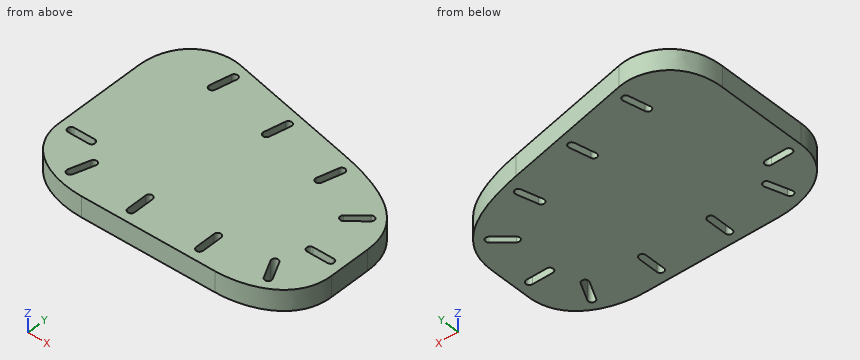
from build123d import *

# Parameters (mm, degrees)
EXTRUDE_1_DEPTH       = 10
CUT_EXTRUDE_1_DEPTH   = 149.427210809
PATTERN_CURVE_1_DEPTH = 10


# Read off the part's stored shape, not the designer's step: Кривая1
with BuildPart() as part:
    # Эскиз1_fr → Бобышка-Вытянуть1 (new body)
    with BuildSketch(Plane.XY):
        with BuildLine():
            Line((0, 0), (0, 20))
            add(Edge.make_bspline(
                [(0, 20), (0, 38.146025899), (-14.209474182, 48.611098897), (-41.986949672, 54.649680525)],
                knots=[0, 0, 0, 0, 1, 1, 1, 1], degree=3))
            Line((-41.986949672, 54.649680525), (-103.301225383, 67.978870897))
            add(Edge.make_bspline(
                [(-103.301225383, 67.978870897), (-115.500001367, 70.63077872), (-131.292525164, 63.393306184), (-131.292525164, 43.097715536)],
                knots=[0, 0, 0, 0, 1, 1, 1, 1], degree=3))
            Line((-131.292525164, 43.097715536), (-131.292525164, 0))
            add(Edge.make_bspline(
                [(-97.969549234, -25.769768053), (-112.011160689, -25.769768053), (-131.292525164, -19.025155818), (-131.292525164, 0)],
                knots=[0, 0, 0, 0, 1, 1, 1, 1], degree=3))
            Line((-97.969549234, -25.769768053), (-33.545129103, -25.769768053))
            add(Edge.make_bspline(
                [(-33.545129103, -25.769768053), (-19.444866568, -25.769768053), (0, -19.063757455), (0, 0)],
                knots=[0, 0, 0, 0, 1, 1, 1, 1], degree=3))
        make_face()
    extrude(amount=EXTRUDE_1_DEPTH)

    # Эскиз2_fr → Вырез-Вытянуть1 (cut, through all)
    with BuildSketch(Plane(origin=(0, 0, 0), x_dir=(-1, 0, 0), z_dir=(0, 0, -1))):
        with BuildLine():
            Line((102.429251955, 61.832882372), (104.527789693, 52.179608775))
            ThreePointArc((104.527789693, 52.179608775), (103.259303337, 50.206407776), (101.286102339, 51.474894133))
            Line((101.286102339, 51.474894133), (99.1875646, 61.128167729))
            ThreePointArc((99.1875646, 61.128167729), (100.456050956, 63.101368728), (102.429251955, 61.832882372))
        make_face()
    extrude(amount=-CUT_EXTRUDE_1_DEPTH, mode=Mode.SUBTRACT)

    # Кривая1 outline → Кривая1 (cut)
    with BuildSketch(Plane.XY):
        with BuildLine():
            ThreePointArc((-66.925496948, 54.114674761), (-68.193983304, 56.08787576), (-70.167184303, 54.819389404))
            Line((-70.167184303, 54.819389404), (-72.265722041, 45.166115807))
            ThreePointArc((-72.265722041, 45.166115807), (-70.997235685, 43.192914809), (-69.024034687, 44.461401165))
            Line((-69.024034687, 44.461401165), (-66.925496948, 54.114674761))
        make_face()
        with BuildLine():
            ThreePointArc((-34.992445024, 46.929960503), (-36.164147849, 48.962124942), (-38.196312288, 47.790422117))
            Line((-38.196312288, 47.790422117), (-40.758641861, 38.249771252))
            ThreePointArc((-40.758641861, 38.249771252), (-39.586939036, 36.217606813), (-37.554774597, 37.389309638))
            Line((-37.554774597, 37.389309638), (-34.992445024, 46.929960503))
        make_face()
        with BuildLine():
            ThreePointArc((-9.659083383, 32.724100966), (-9.478152386, 35.062870683), (-11.816922103, 35.243801681))
            Line((-11.816922103, 35.243801681), (-19.320224464, 28.818071725))
            ThreePointArc((-19.320224464, 28.818071725), (-19.501155461, 26.479302007), (-17.162385743, 26.298371011))
            Line((-17.162385743, 26.298371011), (-9.659083383, 32.724100966))
        make_face()
        with BuildLine():
            ThreePointArc((-5.820481715, 4.607864038), (-4.161780443, 6.266565309), (-5.820481715, 7.925266581))
            Line((-5.820481715, 7.925266581), (-15.699224133, 7.925266581))
            ThreePointArc((-15.699224133, 7.925266581), (-17.357925405, 6.266565309), (-15.699224133, 4.607864038))
            Line((-15.699224133, 4.607864038), (-5.820481715, 4.607864038))
        make_face()
        with BuildLine():
            ThreePointArc((-17.811005152, -16.834920175), (-15.579870133, -17.559224215), (-14.855566092, -15.328089196))
            Line((-14.855566092, -15.328089196), (-19.342689651, -6.527221402))
            ThreePointArc((-19.342689651, -6.527221402), (-21.573824671, -5.802917361), (-22.298128711, -8.034052381))
            Line((-22.298128711, -8.034052381), (-17.811005152, -16.834920175))
        make_face()
        with BuildLine():
            ThreePointArc((-47.67905304, -19.949286338), (-46.020351768, -21.607987609), (-44.361650497, -19.949286338))
            Line((-44.361650497, -19.949286338), (-44.361650497, -10.070543919))
            ThreePointArc((-44.361650497, -10.070543919), (-46.020351768, -8.411842648), (-47.67905304, -10.070543919))
            Line((-47.67905304, -10.070543919), (-47.67905304, -19.949286338))
        make_face()
        with BuildLine():
            ThreePointArc((-80.694656818, -19.949286338), (-79.035955546, -21.607987609), (-77.377254274, -19.949286338))
            Line((-77.377254274, -19.949286338), (-77.377254274, -10.070543919))
            ThreePointArc((-77.377254274, -10.070543919), (-79.035955546, -8.411842648), (-80.694656818, -10.070543919))
            Line((-80.694656818, -10.070543919), (-80.694656818, -19.949286338))
        make_face()
        with BuildLine():
            ThreePointArc((-111.662441641, -17.601639491), (-110.581423079, -19.683460493), (-108.499602077, -18.602441931))
            Line((-108.499602077, -18.602441931), (-105.519357928, -9.18396559))
            ThreePointArc((-105.519357928, -9.18396559), (-106.60037649, -7.102144588), (-108.682197492, -8.18316315))
            Line((-108.682197492, -8.18316315), (-111.662441641, -17.601639491))
        make_face()
        with BuildLine():
            ThreePointArc((-125.472043449, 1.658701272), (-127.130744721, 0), (-125.472043449, -1.658701272))
            Line((-125.472043449, -1.658701272), (-115.593301031, -1.658701272))
            ThreePointArc((-115.593301031, -1.658701272), (-113.934599759, 0), (-115.593301031, 1.658701272))
            Line((-115.593301031, 1.658701272), (-125.472043449, 1.658701272))
        make_face()
    extrude(amount=PATTERN_CURVE_1_DEPTH, mode=Mode.SUBTRACT)


solid = part.part
Source: CAD feature listing. Evaluate the final solid. Frame: model axes, mm. Coordinates: 2 decimals unless noted, no trailing zeros. Loops run counter-clockwise (first coordinate to the right, second up) from the corner with the lowest first, then second, coordinate; pieces in that order, holes last. Notation, with made-up numbers: (87, 81.5) - (138, 81.5) arc R24 cw to (138, 91.5) - close; hole circle Ø4 at (-17, -2.75). An arc over 180 degrees is marked (long way). One line per item, written item: value. Start each with the question number.
1. Section B-B (x = -74.5). Return the cut outline in (y, z), and give its area (3 significant figures).
2. Section C-C (x = -93). Return the cut outline in (y, z), and give its area (3 significant figures).
3. Section A-A (z = 4.5). State how many separate pieces and enclosed holes the cut face has, and give its area (3 significant figures).
4. Contact query for flat-ended pins moving along their axis: P1, Ø3, axis at x = -119, z = 5, coming from the +Y side; P2, Ø5, axis at y = -16, z = 6, coming from the -X side; P3, Ø5, axis at y = -14, z = 3, coming from the +X side. Output: stop coordinate, or through.
5. Ray query, L1, parallel to X at y = -10, z = 0.5; L2, parallel to X at y = -9.5, z = 4; L3, parallel to X at y = 6.5, z = 5. Return the intervals inside material, ascending.
Verdict:
1. outline: (-25.77, 0) - (61.72, 0) - (61.72, 10) - (-25.77, 10) - close
1. area: 875 mm2
2. outline: (-25.77, 0) - (65.74, 0) - (65.74, 10) - (-25.77, 10) - close
2. area: 915 mm2
3. separate pieces: 1
3. enclosed holes: 10
3. area: 10,100 mm2
4. P1: stops at y = 66.63
4. P2: stops at x = -127.09
4. P3: stops at x = -2.92
5. L1: x = -129.17 to -109.26, -105.78 to -80.69, -77.38 to -47.68, -44.36 to -21.3, -17.57 to -2.13
5. L2: x = -129.4 to -109.1, -105.62 to -80.59, -77.48 to -47.58, -44.46 to -21.55, -17.83 to -1.91
5. L3: x = -131.29 to -17.34, -4.18 to 0
